from build123d import *

# Parameters (mm, degrees)
F0_W         = 65.6
F0_H         = 24.2
F0_W_2       = 60.8
F0_H_2       = 19.4
F1_DEPTH     = 10
F2_DEPTH     = 2
F4_DEPTH     = 65.601
F5_W         = 65.6
F5_H         = 20
F6_DEPTH     = 5
F7_R         = 1
F8_R         = 1
F9_T1_DEPTH  = 31.5
F9_T3_DEPTH  = 11.5
F9_S7_W      = 1
F9_S7_H      = 1
F9_T8_DEPTH  = 1
F9_S13_W     = 1
F9_S13_H     = 1
F9_T14_DEPTH = 1
F9_S19_W     = 1
F9_S19_H     = 1
F9_T20_DEPTH = 1
F9_S25_W     = 1
F9_S25_H     = 1
F9_T26_DEPTH = 1


# Not quite as in the source:
# - a fillet or chamfer that OpenCascade refuses, or shapes differently, is made with other operations: its cross-section is extruded or revolved along the edge and cut away or added


with BuildPart() as f1:
    # F0 (on Top) → F1 (new body)
    with BuildSketch(Plane.XY):
        Rectangle(F0_W, F0_H)
        Rectangle(F0_W_2, F0_H_2, mode=Mode.SUBTRACT)
    extrude(amount=F1_DEPTH)

    # F0 (on Top) → F2 (join)
    with BuildSketch(Plane.XY):
        Rectangle(F0_W_2, F0_H_2)
    extrude(amount=F2_DEPTH)

    # F3 (on face) → F4 (cut, through all)
    with BuildSketch(Plane.YZ.offset(32.8)):
        Polygon((2.2, 10), (0, 10), (-2.2, 10), (-2.2, 4.5), (0, 4.5), (2.2, 4.5), align=None)
    extrude(amount=-F4_DEPTH, mode=Mode.SUBTRACT)

    # F5 (on face) → F6 (join)
    with BuildSketch(Plane(origin=(0, 12.1, 0), x_dir=(-1, 0, 0), z_dir=(0, 1, 0))):
        with Locations((0, -10)):
            Rectangle(F5_W, F5_H)
    extrude(amount=-F6_DEPTH)

    # F7
    f7_edges = [f1.edges().sort_by_distance(p)[0] for p in [
        (0, -9.7, 10),
        (0, -12.1, 10),
        (-32.8, -7.15, 10),
        (32.8, -7.15, 10),
        (30.4, -5.95, 10),
        (-31.6, -2.2, 10),
        (31.6, -2.2, 10),
        (-30.4, -5.95, 10),
    ]]
    fillet(f7_edges, radius=F7_R)

    # F8
    f8_edges = [f1.edges().sort_by_distance(p)[0] for p in [
        (-31.6, 2.2, 10),
        (31.6, 2.2, 10),
        (32.8, 7.15, 10),
        (-32.8, 7.15, 10),
        (-30.4, 5.95, 10),
        (30.4, 5.95, 10),
        (0, 9.7, 10),
        (0, 12.1, 10),
    ]]
    fillet(f8_edges, radius=F8_R)

    # F9: fillet of radius 1 on 4 edges, made by hand

    # F9_s2 → F9_t1 (cut)
    with BuildSketch(Plane.XY.offset(-22.5)):
        with BuildLine():
            ThreePointArc((31.8, 12.1), (32.5071067812, 11.8071067812), (32.8, 11.1))
            Line((32.8, 11.1), (32.8, 12.1))
            Line((32.8, 12.1), (31.8, 12.1))
        make_face()
        with BuildLine():
            ThreePointArc((-32.8, 11.1), (-32.5071067812, 11.8071067812), (-31.8, 12.1))
            Line((-31.8, 12.1), (-32.8, 12.1))
            Line((-32.8, 12.1), (-32.8, 11.1))
        make_face()
    extrude(amount=F9_T1_DEPTH, mode=Mode.SUBTRACT)

    # F9_s4 → F9_t3 (cut)
    with BuildSketch(Plane.XY.offset(-2.5)):
        with BuildLine():
            ThreePointArc((31.8, -12.1), (32.5071067812, -11.8071067812), (32.8, -11.1))
            Line((32.8, -11.1), (32.8, -12.1))
            Line((32.8, -12.1), (31.8, -12.1))
        make_face()
        with BuildLine():
            ThreePointArc((-32.8, -11.1), (-32.5071067812, -11.8071067812), (-31.8, -12.1))
            Line((-31.8, -12.1), (-32.8, -12.1))
            Line((-32.8, -12.1), (-32.8, -11.1))
        make_face()
    extrude(amount=F9_T3_DEPTH, mode=Mode.SUBTRACT)


with BuildPart() as f9_tool6:
    # F9_s7 → F9_t8 (new body)
    with BuildSketch(Plane.YZ.offset(-31.8)):
        with Locations((-11.6, 9.5)):
            Rectangle(F9_S7_W, F9_S7_H)
    extrude(amount=-F9_T8_DEPTH)

    # F9_s9 → F9_t10 (revolve, cut)
    with BuildSketch(Plane(origin=(-31.8, -11.1, 9), x_dir=(0, 0.7071067812, -0.7071067812), z_dir=(0, 0.7071067812, 0.7071067812))):
        with BuildLine():
            ThreePointArc((0, -1), (1, 0), (0, 1))
            Line((0, 1), (0, -1))
        make_face()
    revolve(axis=Axis((-31.8, -11.1, 9), (-1, 0, 0)), mode=Mode.SUBTRACT)


with BuildPart() as f1_1:
    add(f1.part)

    # F9_t5: cut F9_tool6
    add(f9_tool6.part, mode=Mode.SUBTRACT)


with BuildPart() as f9_tool12:
    # F9_s13 → F9_t14 (new body)
    with BuildSketch(Plane.YZ.offset(-31.8)):
        with Locations((11.6, 9.5)):
            Rectangle(F9_S13_W, F9_S13_H)
    extrude(amount=-F9_T14_DEPTH)

    # F9_s15 → F9_t16 (revolve, cut)
    with BuildSketch(Plane(origin=(-31.8, 11.1, 9), x_dir=(0, -0.7071067812, -0.7071067812), z_dir=(0, 0.7071067812, -0.7071067812))):
        with BuildLine():
            ThreePointArc((0, -1), (1, 0), (0, 1))
            Line((0, 1), (0, -1))
        make_face()
    revolve(axis=Axis((-31.8, 11.1, 9), (-1, 0, 0)), mode=Mode.SUBTRACT)


with BuildPart() as f1_2:
    add(f1_1.part)

    # F9_t11: cut F9_tool12
    add(f9_tool12.part, mode=Mode.SUBTRACT)


with BuildPart() as f9_tool18:
    # F9_s19 → F9_t20 (new body)
    with BuildSketch(Plane.XZ.offset(11.1)):
        with Locations((32.3, 9.5)):
            Rectangle(F9_S19_W, F9_S19_H)
    extrude(amount=F9_T20_DEPTH)

    # F9_s21 → F9_t22 (revolve, cut)
    with BuildSketch(Plane(origin=(31.8, -11.1, 9), x_dir=(-0.7071067812, 0, -0.7071067812), z_dir=(-0.7071067812, 0, 0.7071067812))):
        with BuildLine():
            ThreePointArc((0, -1), (1, 0), (0, 1))
            Line((0, 1), (0, -1))
        make_face()
    revolve(axis=Axis((31.8, -11.1, 9), (0, -1, 0)), mode=Mode.SUBTRACT)


with BuildPart() as f1_3:
    add(f1_2.part)

    # F9_t17: cut F9_tool18
    add(f9_tool18.part, mode=Mode.SUBTRACT)


with BuildPart() as f9_tool24:
    # F9_s25 → F9_t26 (new body)
    with BuildSketch(Plane.XZ.offset(-11.1)):
        with Locations((32.3, 9.5)):
            Rectangle(F9_S25_W, F9_S25_H)
    extrude(amount=-F9_T26_DEPTH)

    # F9_s27 → F9_t28 (revolve, cut)
    with BuildSketch(Plane(origin=(31.8, 11.1, 9), x_dir=(-0.7071067812, 0, -0.7071067812), z_dir=(0.7071067812, 0, -0.7071067812))):
        with BuildLine():
            ThreePointArc((0, -1), (1, 0), (0, 1))
            Line((0, 1), (0, -1))
        make_face()
    revolve(axis=Axis((31.8, 11.1, 9), (0, 1, 0)), mode=Mode.SUBTRACT)


with BuildPart() as f1_4:
    add(f1_3.part)

    # F9_t23: cut F9_tool24
    add(f9_tool24.part, mode=Mode.SUBTRACT)


solid = f1_4.part
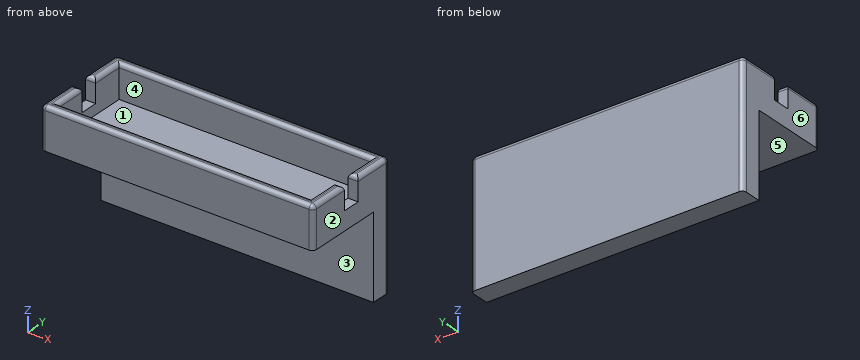
Model file for the job. Use its own axes, mm. Face numbers are marked on the shaded views. A direction names the side the tool comes from. Give positions to 0.01 mm unless a question says otherwise; leave off trailing zeros. Loops run counter-clockwise (first coordinate to the right, second up) from the corner with the lowest first, then second, coordinate; pieces in that order, holes last. Notation, with made-up numbers: (81.25, -26.5) -> (87.25, -26.5) arc R15 ccw to (87.25, -21.5) -> close; hole circle Ø10 at (44, 53). An arc over 180 degrees is marked (long way). Use a Markdown table: item, result. Add a question column.
(1) Slice it at D-D on z = -5.75. List the corners of the cut face in (x, y), and give its area (3 significant figures).
(2) Slice it at C-C on x = -9. List the corners of the cut face in (y, z).
(3) Slice it at B-B on y = 1.5. List the corners of the cut face in (x, z), and give its area (3 significant figures).
(4) Tool access for the marked faces 4, 5 and 6: list every direction of +Z, -Z, +X, -X, +Y, -Y with a clear straight run to the whole face (end or side of a thin tool).
(5) Mould opens along Y. For the marked faces 1, 2 and 3 say: +Y half, -Y half, draft (parallel to the pull), parting line (faces both ways), or undercut.
(6) Slice it at A-A on z = 6.5. List the corners of the cut face in (x, y), and give its area (3 significant figures).
(7) Drop flat-ended pins along their axis: pin 1 Ø2 at (x, y) = (-8, 9) entering from +Z; pin 2 Ø3 at (x, y) = (23, -3) entering from +Z; pin 3 Ø1.9 at (x, y) = (-31.5, 1) entering from +Z. Give the stop position or say it passes through.
(8) Wall check: line 1 along Y through (x, z) = (-29.5, 3.75); line 2 along Z through (x, y) = (-15, 6.25); line 3 along Y through (x, z) = (25.5, -2.5). Give the ranges that are in metal, low to high.
Filled sheet:
| question | item | result |
|---|---|---|
| 1 | outline | (-32.8, 7.1) -> (32.8, 7.1) -> (32.8, 11.1) arc R1 ccw to (31.8, 12.1) -> (-31.8, 12.1) arc R1 ccw to (-32.8, 11.1) -> close |
| 1 | area | 328 mm2 |
| 2 | outline | (-12.1, 0) -> (7.1, 0) -> (7.1, -20) -> (12.1, -20) -> (12.1, 9) arc R1 ccw to (11.1, 10) -> (10.7, 10) arc R1 ccw to (9.7, 9) -> (9.7, 2) -> (-9.7, 2) -> (-9.7, 9) arc R1 ccw to (-10.7, 10) -> (-11.1, 10) arc R1 ccw to (-12.1, 9) -> close |
| 3 | outline | (-32.8, 0) -> (32.8, 0) -> (32.8, 4.5) -> (30.4, 4.5) -> (30.4, 2) -> (-30.4, 2) -> (-30.4, 4.5) -> (-32.8, 4.5) -> close |
| 3 | area | 143 mm2 |
| 4 | face 4 | +Z |
| 4 | face 5 | -Z, +X, -X, -Y |
| 4 | face 6 | +Z, -Z, -X, +Y, -Y |
| 5 | face 1 | undercut |
| 5 | face 2 | draft |
| 5 | face 3 | -Y half |
| 6 | outline | (-32.8, -11.1) arc R1 ccw to (-31.8, -12.1) -> (31.8, -12.1) arc R1 ccw to (32.8, -11.1) -> (32.8, -2.2) -> (30.4, -2.2) -> (30.4, -9.7) -> (-30.4, -9.7) -> (-30.4, -2.2) -> (-32.8, -2.2) -> close; (-32.8, 2.2) -> (-30.4, 2.2) -> (-30.4, 9.7) -> (30.4, 9.7) -> (30.4, 2.2) -> (32.8, 2.2) -> (32.8, 11.1) arc R1 ccw to (31.8, 12.1) -> (-31.8, 12.1) arc R1 ccw to (-32.8, 11.1) -> close |
| 6 | area | 386 mm2 |
| 7 | pin 1 | z = 9.71 |
| 7 | pin 2 | z = 2 |
| 7 | pin 3 | z = 4.5 |
| 8 | line 1 | -12.1 to -9.7, 9.7 to 12.1 |
| 8 | line 2 | 0 to 2 |
| 8 | line 3 | 7.1 to 12.1 |
